Source: three-view drawing plus pictorial views. Frame: mm from the lowest corner of the part. Round coordinates to 2 decimals unless told otherwise and drop trailing zeros. Write each loop counter-clockwise with the first axis right and the second up, starting at its lowest first coordinate (ties: lowest second). Pieces come first, ordered by that corner, then holes. Notation, with made-up numbers: M 87,56 L 95,56 A22 cw 95,66 Z; hole C -2.5,87 d11. An arc over 180 degrees is marked long. Put each result on its own line as item: value. Start each with the question number.
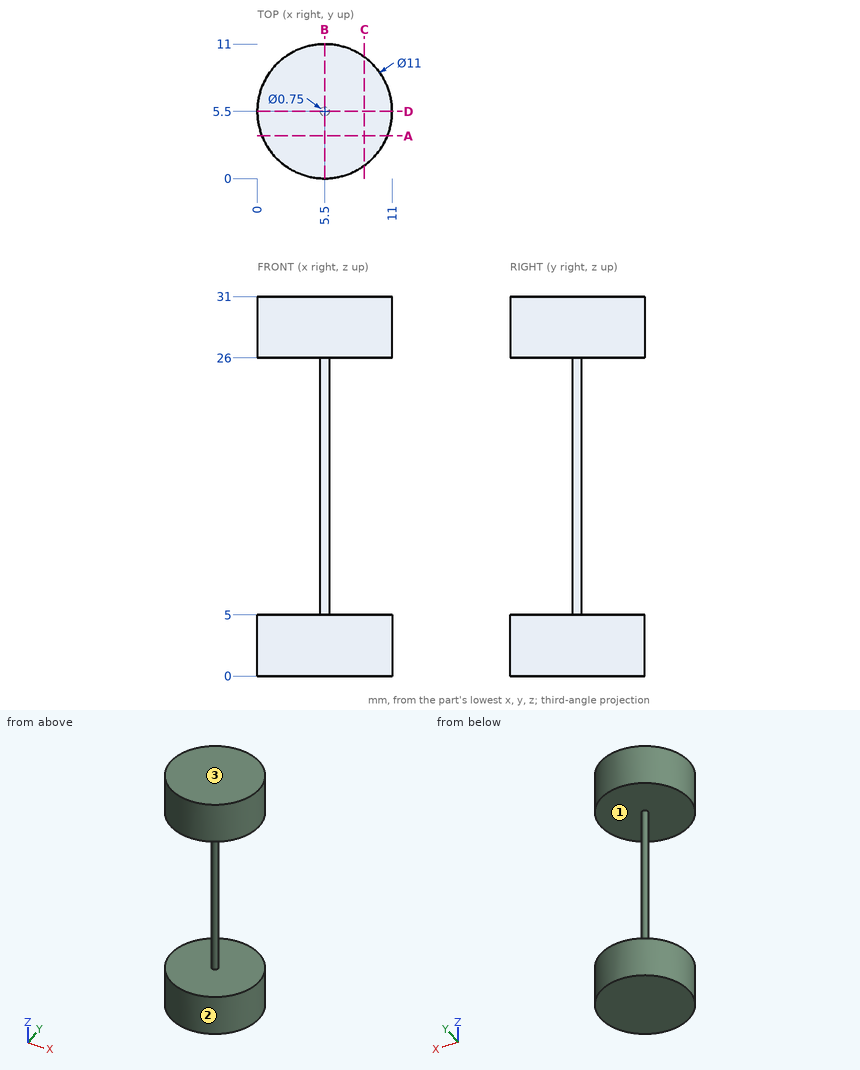
(1) Pull-direction query (Z, two-part tool) for the marked faces 1, 2 and 3; classes: +Z half, -Z half, draft (parallel to the pull), parting line (faces both ways), or undercut.
(2) Section query B-B (x = 5.5). Return loops of the section in (y, z) (3 decimals), and give its area (3 significant figures).
(3) Section query C-C (x = 8.75). Return loops of the section in (y, z), and give its area (3 significant figures).
(4) Ray query, line 1 along Z through (x, y) = (9.75, 4.5); line 2 along X through (y, z) = (7.25, 29); line 3 along Y through (x, z) = (5, 28.5). Return the intervals inside material, ascending.
(5) Contact query for flat-ended pins moving along their axis: P1, Ø4, axis at y = 6, z = 17, coming from the -X side (3 decimals); P2, Ø6, axis at x = 9, z = 26, coming from the +Y side. Output: stop coordinate, or through.
(6) Section query A-A (y = 3.5). Return loops of the section in (x, z), and give its area (3 significant figures).
Entries:
1. face 1: undercut
1. face 2: draft
1. face 3: +Z half
2. outline: M 0,0 L 11,0 L 11,5 L 5.875,5 L 5.875,26 L 11,26 L 11,31 L 0,31 L 0,26 L 5.125,26 L 5.125,5 L 0,5 Z
2. area: 126 mm2
3. outline: M 1.06,0 L 9.94,0 L 9.94,5 L 1.06,5 Z; M 1.06,26 L 9.94,26 L 9.94,31 L 1.06,31 Z
3. area: 88.7 mm2
4. line 1: 0 to 5, 26 to 31
4. line 2: 0.29 to 10.71
4. line 3: 0.02 to 10.98
5. P1: x = 5.125
5. P2: y = 10.98
6. outline: M 0.38,0 L 10.62,0 L 10.62,5 L 0.38,5 Z; M 0.38,26 L 10.62,26 L 10.62,31 L 0.38,31 Z
6. area: 102 mm2
